The model under review builds one solid part; all positions refer to its coordinate system, in mm. Give positions to 0.01 mm unless a question says otherwise; leave off trailing zeros. Loops run counter-clockwise (first coordinate to the right, second up) from the corner with the lowest first, then second, coordinate; pieces in that order, holes last. Notation, with made-up numbers: M 24.25,79 L 63.25,79 A13 ccw 63.25,91 Z; hole C 39.25,1.5 d4. An arc over 180 degrees is marked long. Put each result on its own line as item: value. Start each with the question number.
```python
from build123d import *

# Parameters (mm, degrees)
SKETCH1_R           = 0.5
BOSS_EXTRUDE1_DEPTH = 0.5


with BuildPart() as part:
    # Sketch1 → Boss-Extrude1 (new body)
    with BuildSketch(Plane(origin=(0, 0, 0), x_dir=(1, 0, 0), z_dir=(0, 1, 0))):
        with BuildLine():
            Line((6.155, 2.9), (10.255, 2.9))
            ThreePointArc((10.255, 2.9), (10.608553391, 2.753553391), (10.755, 2.4))
            Line((10.755, 2.4), (10.755, -2.4))
            ThreePointArc((10.755, -2.4), (10.608553391, -2.753553391), (10.255, -2.9))
            Line((10.255, -2.9), (-6.445, -2.9))
            ThreePointArc((-6.445, -2.9), (-6.798553391, -2.753553391), (-6.945, -2.4))
            Line((-6.945, -2.4), (-6.945, 2.4))
            ThreePointArc((-6.945, 2.4), (-6.798553391, 2.753553391), (-6.445, 2.9))
            Line((-6.445, 2.9), (-2.345, 2.9))
            Line((-2.345, 2.9), (-2.345, 4.1))
            Line((-2.345, 4.1), (6.155, 4.1))
            Line((6.155, 4.1), (6.155, 2.9))
        make_face()
        with Locations(Location((0, 0, 0), (0, 0, 270))):
            Circle(SKETCH1_R, mode=Mode.SUBTRACT)
        with Locations(Location((3.81, 0, 0), (0, 0, 270))):
            Circle(SKETCH1_R, mode=Mode.SUBTRACT)
    extrude(amount=BOSS_EXTRUDE1_DEPTH)


solid = part.part
```
Item 1: Consider section B-B, the plane x = 3.81. Write out the cut boundary in (y, z).
Item 2: Draft analysis for pull direction X (two halves, no side actions). For faces 1 (the flat face through (2, 0, -1)), 2 (the cylindrical face through (4.3, 0.2, -0.1)), state which applies: +X half, -X half, draft (parallel to the pull), parting line (faces both ways), or undercut.
Item 3: Consider section A-A, the plane z = 0. Write out the cut boundary in (x, y) (3 decimals), plus the area to 3 significant figures.
Item 4: To check wall thickness, follow L1, parallel to X at y = 0.45, z = 0 (3 decimals); L2, parallel to Z at x = -3.75, y = 0.1; L3, parallel to Z at x = -0.25, y = 0.1. State the ranges of each line that lie inside material, in increasing order. Write a range as [from, to].
Item 5: Consider section C-C, the plane y = 0.2. Write out the cut boundary in (x, z) (3 decimals), plus the area to 3 significant figures.
Item 6: Consider section D-D, the plane x = 7.75. Write out the cut boundary in (y, z).
Report:
1. outline: M 0,-4.1 L 0.5,-4.1 L 0.5,-0.5 L 0,-0.5 Z; M 0,0.5 L 0.5,0.5 L 0.5,2.9 L 0,2.9 Z
2. face 1: draft
2. face 2: undercut
3. outline: M -6.945,0 L -0.5,0 L -0.5,0.5 L -6.945,0.5 Z; M 0.5,0 L 3.31,0 L 3.31,0.5 L 0.5,0.5 Z; M 4.31,0 L 10.755,0 L 10.755,0.5 L 4.31,0.5 Z
3. area: 7.85 mm²
4. L1: [-6.945, -0.5], [0.5, 3.31], [4.31, 10.755]
4. L2: [-2.9, 2.9]
4. L3: [-4.1, -0.43], [0.43, 2.9]
5. outline: M -6.945,-2.4 A0.5 ccw -6.445,-2.9 L -2.345,-2.9 L -2.345,-4.1 L 6.155,-4.1 L 6.155,-2.9 L 10.255,-2.9 A0.5 ccw 10.755,-2.4 L 10.755,2.4 A0.5 ccw 10.255,2.9 L -6.445,2.9 A0.5 ccw -6.945,2.4 Z; hole C 0,0 d1; hole C 3.81,0 d1
5. area: 111 mm²
6. outline: M 0,-2.9 L 0.5,-2.9 L 0.5,2.9 L 0,2.9 Z
